Can you work these out from the model? Positions are in its coordinate system, mm. A direction names the side the tool comes from. Give positions to 0.01 mm unless a question says otherwise; leave off trailing zeros. Order: outer loops, then holes, each group sorted by start corner. A loop starts at its lowest first (then second) coordinate and runs counter-clockwise, first axis right, second up. Notation, with made-up numbers: M 48,-12 L 78,-12 A11 ccw 78,-3 Z; hole C 25.25,-26 d6. An arc over 180 degrees is marked long. Use a Markdown table: item, result. Add a question column.
from build123d import *

# Parameters (mm, degrees)
F0_R      = 43
F1_DEPTH  = 61
F2_R      = 7.5
F3_DEPTH  = 7.5
F5_DEPTH  = 5
F6_R      = 5
F7_R      = 2.75
F8_DEPTH  = 66.001
F9_R      = 36.5
F9_R_2    = 7.5
F10_DEPTH = 2
F11_R     = 6
F12_DEPTH = 31
F14_DEPTH = 16
F15_R     = 6.5
F15_R_2   = 5
F16_DEPTH = 1


with BuildPart() as f1:
    # F0 (on Front) → F1 (new body)
    with BuildSketch(Plane.XZ):
        Circle(F0_R)
    extrude(amount=F1_DEPTH)

    # F2 (on face) → F3 (cut)
    with BuildSketch(Plane(origin=(0, 0, 0), x_dir=(-1, 0, 0), z_dir=(0, 1, 0))):
        Circle(F2_R)
    extrude(amount=-F3_DEPTH, mode=Mode.SUBTRACT)

    # F4 (on face) → F5 (join)
    with BuildSketch(Plane.XZ.offset(61)):
        with BuildLine():
            Line((-41.25, -12.142384), (-41.25, -41.25))
            Line((-41.25, -41.25), (-12.142384, -41.25))
            ThreePointArc((-12.142384, -41.25), (-30.405592, -30.405592), (-41.25, -12.142384))
        make_face()
        with BuildLine():
            ThreePointArc((-41.25, -12.142384), (-30.405592, -30.405592), (-12.142384, -41.25))
            ThreePointArc((-12.142384, -41.25), (0, -43), (12.142384, -41.25))
            ThreePointArc((12.142384, -41.25), (30.405592, -30.405592), (41.25, -12.142384))
            ThreePointArc((41.25, -12.142384), (42.560251, -6.133922), (43, 0))
            ThreePointArc((43, 0), (42.560251, 6.133922), (41.25, 12.142384))
            ThreePointArc((41.25, 12.142384), (30.405592, 30.405592), (12.142384, 41.25))
            ThreePointArc((12.142384, 41.25), (0, 43), (-12.142384, 41.25))
            ThreePointArc((-12.142384, 41.25), (-30.405592, 30.405592), (-41.25, 12.142384))
            ThreePointArc((-41.25, 12.142384), (-43, 0), (-41.25, -12.142384))
        make_face()
        with BuildLine():
            ThreePointArc((41.25, -12.142384), (30.405592, -30.405592), (12.142384, -41.25))
            Line((12.142384, -41.25), (41.25, -41.25))
            Line((41.25, -41.25), (41.25, -12.142384))
        make_face()
        with BuildLine():
            Line((-41.25, 41.25), (-41.25, 12.142384))
            ThreePointArc((-41.25, 12.142384), (-30.405592, 30.405592), (-12.142384, 41.25))
            Line((-12.142384, 41.25), (-41.25, 41.25))
        make_face()
        with BuildLine():
            Line((41.25, 41.25), (12.142384, 41.25))
            ThreePointArc((12.142384, 41.25), (30.405592, 30.405592), (41.25, 12.142384))
            Line((41.25, 12.142384), (41.25, 41.25))
        make_face()
    extrude(amount=F5_DEPTH)

    # F6
    f6_edges = [f1.edges().sort_by_distance(p)[0] for p in [
        (41.25, -63.5, -41.25),
        (-41.25, -63.5, -41.25),
        (-41.25, -63.5, 41.25),
        (41.25, -63.5, 41.25),
    ]]
    fillet(f6_edges, radius=F6_R)

    # F7 (on face) → F8 (cut, through all)
    with BuildSketch(Plane.XZ.offset(66)):
        with Locations((-34.8, 34.8)):
            Circle(F7_R)
        with Locations((34.8, 34.8)):
            Circle(F7_R)
        with Locations((34.8, -34.8)):
            Circle(F7_R)
        with Locations((-34.8, -34.8)):
            Circle(F7_R)
    extrude(amount=-F8_DEPTH, mode=Mode.SUBTRACT)

    # F9 (on face) → F10 (join)
    with BuildSketch(Plane.XZ.offset(66)):
        Circle(F9_R)
        Circle(F9_R_2, mode=Mode.SUBTRACT)
    extrude(amount=F10_DEPTH)

    # F11 (on face) → F12 (join)
    with BuildSketch(Plane.XZ.offset(66)):
        Circle(F11_R)
    extrude(amount=F12_DEPTH)

    # F13 (on face) → F14 (join)
    with BuildSketch(Plane(origin=(0, 0, 0), x_dir=(-1, 0, 0), z_dir=(0, 1, 0))):
        with BuildLine():
            Line((-18.5, 44.100001), (-18.5, 38.816878))
            ThreePointArc((-18.5, 38.816878), (0, 43), (18.5, 38.816878))
            Line((18.5, 38.816878), (18.5, 44.100001))
            Line((18.5, 44.100001), (14, 51))
            Line((14, 51), (0, 51))
            Line((0, 51), (-14, 51))
            Line((-14, 51), (-18.5, 44.100001))
        make_face()
    extrude(amount=-F14_DEPTH)

    # F15 (on face) → F16 (join)
    with BuildSketch(Plane.XY.offset(51)):
        with Locations((0, -8)):
            Circle(F15_R)
        with Locations((0, -8)):
            Circle(F15_R_2, mode=Mode.SUBTRACT)
    extrude(amount=F16_DEPTH)


solid = f1.part
1. If we section it at A-A, the plane y = -62.5: List the corners of the cut face in (x, z) for me.
2. We'd pull the mould along Z, two halves only. Please class faces 5 (the face through (-39.82, -63.54, 39.75)), 6 (the face through (-7.912, -66.986, -35.632)), 7 (the face through (0, -7.5, 0)): +Z half, -Z half, draft (parallel to the pull), parting line (faces both ways), or undercut.
3. On a 3-axis mill with a long thin cutter (end or side, diameter ignored), from which of +Z, -Z, +X, -X, +Y, -Y can I reach the whole of each face in a straight line? I mean faces 1 (the face through (0, -8, 51)), 2 (the face through (33, -61, -32)), 3 (the face through (38, -66, 1)), 4 (the face through (-18.5, -8, 41)). Say none if no direction works.
4. Will these pins go through, and if not, where does the flat tip stop? pin 1 (6 mm diameter, centred on x = 13.5, y = -31.5, fed in from +Z); pin 2 (4 mm diameter, centred on y = -62.5, z = 22, fed in from +X); pin 3 (9.5 mm diameter, centred on x = -4, z = 46.5, fed in from -Y); pin 4 (3.5 mm diameter, centred on x = -34.8, z = -34.8, fed in from +Y).
5. If we section it at D-D, the plane z = -20: List the corners of the cut face in (x, y) for me.
6. If we section it at C-C, the plane x = 34.8: List the corners of the cut face in (y, z) for me.
7. I need wall thicknesses on L1, parallel to Y at x = 0, z = 51.7; L2, parallel to Y at x = 32, z = 5.5; L3, parallel to Y at x = -38, z = 14. Which ranges of each line are inside material? Lowest first, please. Write a range as [from, to].
Geometry results:
| question | item | result |
|---|---|---|
| 1 | outline | M -41.25,-36.25 A5 ccw -36.25,-41.25 L -12.14,-41.25 A43 ccw 12.14,-41.25 L 36.25,-41.25 A5 ccw 41.25,-36.25 L 41.25,-12.14 A43 ccw 43,0 A43 ccw 41.25,12.14 L 41.25,36.25 A5 ccw 36.25,41.25 L 12.14,41.25 A43 ccw -12.14,41.25 L -36.25,41.25 A5 ccw -41.25,36.25 L -41.25,12.14 A43 ccw -41.25,-12.14 Z; hole C -34.8,-34.8 d5.5; hole C -34.8,34.8 d5.5; hole C 34.8,-34.8 d5.5; hole C 34.8,34.8 d5.5 |
| 2 | face 5 | +Z half |
| 2 | face 6 | parting line |
| 2 | face 7 | undercut |
| 3 | face 1 | +Z |
| 3 | face 2 | -Z, +X, +Y |
| 3 | face 3 | -Y |
| 3 | face 4 | +Z, -X, +Y |
| 4 | pin 1 | stops at z = 41.7 |
| 4 | pin 2 | stops at x = 41.25 |
| 4 | pin 3 | stops at y = -66 |
| 4 | pin 4 | passes through |
| 5 | outline | M -41.25,-66 L -30.53,-66 L -30.53,-68 L 30.53,-68 L 30.53,-66 L 41.25,-66 L 41.25,-61 L 38.07,-61 L 38.07,0 L -38.07,0 L -38.07,-61 L -41.25,-61 Z |
| 6 | outline | M -68,-11.01 L -66,-11.01 L -66,-32.05 L -61,-32.05 L -61,-25.26 L 0,-25.26 L 0,25.26 L -61,25.26 L -61,32.05 L -66,32.05 L -66,11.01 L -68,11.01 Z; M -66,-41.25 L -61,-41.25 L -61,-37.55 L -66,-37.55 Z; M -66,37.55 L -61,37.55 L -61,41.25 L -66,41.25 Z |
| 7 | L1 | y = [-14.5, -13], [-3, -1.5] |
| 7 | L2 | y = [-68, 0] |
| 7 | L3 | y = [-66, 0] |
